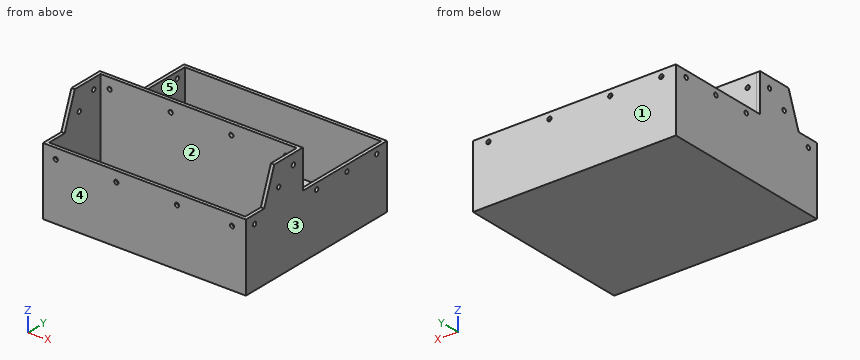
```python
from build123d import *

# Parameters (mm, degrees)
SKETCH1_W           = 190.5
SKETCH1_H           = 166.116
BOSS_EXTRUDE1_DEPTH = 95.25
CUT_EXTRUDE1_DEPTH  = 92.075
CUT_EXTRUDE5_DEPTH  = 35.98418
SKETCH17_W          = 190.5
SKETCH17_H          = 33.474363619
CUT_EXTRUDE6_DEPTH  = 31.75
BOSS_EXTRUDE8_DEPTH = 190.5
SKETCH19_W          = 184.15
SKETCH19_H          = 30.313503047
CUT_EXTRUDE7_DEPTH  = 92.075
SKETCH20_W          = 184.15
SKETCH20_H          = 33.914711244
CUT_EXTRUDE8_DEPTH  = 13.175
CUT_EXTRUDE9_DEPTH  = 60.325
SKETCH23_R          = 2.00000108
CUT_EXTRUDE10_DEPTH = 2.54
SKETCH24_R          = 2
SKETCH24_R_2        = 2.00000108
CUT_EXTRUDE11_DEPTH = 2.54
SKETCH25_R          = 2.00000108
CUT_EXTRUDE12_DEPTH = 229.607619873
SKETCH27_R          = 2.00000108
CUT_EXTRUDE13_DEPTH = 3.175
SKETCH28_R          = 2.00000108
CUT_EXTRUDE15_DEPTH = 229.607619873


with BuildPart() as part:
    # Sketch1 → Boss-Extrude1 (new body)
    with BuildSketch(Plane.XY):
        Rectangle(SKETCH1_W, SKETCH1_H)
    extrude(amount=BOSS_EXTRUDE1_DEPTH)

    # Sketch3 → Cut-Extrude1 (cut)
    with BuildSketch(Plane.XY.offset(95.25)):
        Polygon((-92.075, 79.883), (-92.075, 32.891702926), (-92.075, -16.095133334), (92.075, -16.095133334), (92.075, 48.662739539), (92.075, 79.883), (83.88326961, 79.883), (-81.085829842, 79.883), align=None)
    extrude(amount=-CUT_EXTRUDE1_DEPTH, mode=Mode.SUBTRACT)

    # Sketch15 → Cut-Extrude5 (cut)
    with BuildSketch(Plane.XY.offset(95.25)):
        Polygon((95.25, -16.109272762), (95.25, 83.058), (-95.25, 83.058), (-95.25, -16.109272762), (-92.075, -16.095133334), (-92.075, 79.883), (92.075, 79.883), (92.075, -16.095133334), align=None)
    extrude(amount=-CUT_EXTRUDE5_DEPTH, mode=Mode.SUBTRACT)

    # Sketch17 → Cut-Extrude6 (cut)
    with BuildSketch(Plane.XY.offset(95.25)):
        with Locations((0, -66.320818191)):
            Rectangle(SKETCH17_W, SKETCH17_H)
    extrude(amount=-CUT_EXTRUDE6_DEPTH, mode=Mode.SUBTRACT)

    # Sketch18 → Boss-Extrude8 (add)
    with BuildSketch(Plane.ZY.offset(95.25)):
        Polygon((63.5, -49.583636381), (63.5, -61.506100001), (95.25, -49.583636381), align=None)
    extrude(amount=-BOSS_EXTRUDE8_DEPTH)

    # Sketch19 → Cut-Extrude7 (cut)
    with BuildSketch(Plane.XY.offset(95.25)):
        with Locations((0, -34.426884857)):
            Rectangle(SKETCH19_W, SKETCH19_H)
    extrude(amount=-CUT_EXTRUDE7_DEPTH, mode=Mode.SUBTRACT)

    # Sketch20 → Cut-Extrude8 (cut)
    with BuildSketch(Plane(origin=(0, -74.803163357, 28.08938563), x_dir=(1, 0, 0), z_dir=(0, -0.9361719099317519, 0.3515425366221503))):
        with Locations((0, 54.782261491)):
            Rectangle(SKETCH20_W, SKETCH20_H)
    extrude(amount=-CUT_EXTRUDE8_DEPTH, mode=Mode.SUBTRACT)

    # Sketch21 → Cut-Extrude9 (cut)
    with BuildSketch(Plane.XY.offset(63.5)):
        Polygon((-92.075, -61.506100001), (-92.075, -49.583636381), (92.075, -49.583636381), (92.075, -61.506100001), (92.075, -79.883), (-92.075, -79.883), align=None)
    extrude(amount=-CUT_EXTRUDE9_DEPTH, mode=Mode.SUBTRACT)

    # Sketch23 → Cut-Extrude10 (cut)
    with BuildSketch(Plane.XZ.offset(83.058)):
        with Locations(Location((-83.319719804, 53.848, 0), (0, 0, 270))):
            Circle(SKETCH23_R)
        with Locations(Location((-26.423719804, 53.848, 0), (0, 0, 270))):
            Circle(SKETCH23_R)
        with Locations(Location((30.472280196, 53.848, 0), (0, 0, 270))):
            Circle(SKETCH23_R)
        with Locations(Location((82.288280196, 53.848, 0), (0, 0, 270))):
            Circle(SKETCH23_R)
    extrude(amount=-CUT_EXTRUDE10_DEPTH, mode=Mode.SUBTRACT)

    # Sketch24 → Cut-Extrude11 (cut)
    with BuildSketch(Plane(origin=(0, 83.058, 0), x_dir=(1, 0, 0), z_dir=(0, 1, 0))):
        with Locations(Location((80.65616897, -53.55082, 0), (0, 0, 270))):
            Circle(SKETCH24_R)
        with Locations(Location((23.50616897, -53.55082, 0), (0, 0, 270))):
            Circle(SKETCH24_R_2)
        with Locations(Location((-33.64383103, -53.55082, 0), (0, 0, 270))):
            Circle(SKETCH24_R_2)
        with Locations(Location((-81.568772043, -53.55082, 0), (0, 0, 270))):
            Circle(SKETCH24_R_2)
    extrude(amount=-CUT_EXTRUDE11_DEPTH, mode=Mode.SUBTRACT)

    # Sketch25 → Cut-Extrude12 (cut, through all)
    with BuildSketch(Plane(origin=(95.25, 0, 0), x_dir=(0, 0, -1), z_dir=(1, 0, 0))):
        with Locations((-53.42382, 70.993)):
            Circle(SKETCH25_R)
        with Locations((-53.42382, 35.941)):
            Circle(SKETCH25_R)
        with Locations((-53.42382, 0.217760577)):
            Circle(SKETCH25_R)
    extrude(amount=-CUT_EXTRUDE12_DEPTH, mode=Mode.SUBTRACT)

    # Sketch27 → Cut-Extrude13 (cut)
    with BuildSketch(Plane(origin=(0, -16.095133334, 0), x_dir=(1, 0, 0), z_dir=(0, 1, 0))):
        with Locations(Location((82.042, -85.344, 0), (0, 0, 270))):
            Circle(SKETCH27_R)
        with Locations(Location((30.734, -85.344, 0), (0, 0, 270))):
            Circle(SKETCH27_R)
        with Locations(Location((-26.268567804, -85.344, 0), (0, 0, 270))):
            Circle(SKETCH27_R)
        with Locations(Location((-83.566, -85.344, 0), (0, 0, 270))):
            Circle(SKETCH27_R)
    extrude(amount=-CUT_EXTRUDE13_DEPTH, mode=Mode.SUBTRACT)

    # Sketch28 → Cut-Extrude15 (cut, through all)
    with BuildSketch(Plane(origin=(95.25, 0, 0), x_dir=(0, 0, -1), z_dir=(1, 0, 0))):
        with Locations((-55.372, -72.898)):
            Circle(SKETCH28_R)
        with Locations((-74.422, -44.381878841)):
            Circle(SKETCH28_R)
        with Locations((-85.598, -27.204003713)):
            Circle(SKETCH28_R)
    extrude(amount=-CUT_EXTRUDE15_DEPTH, mode=Mode.SUBTRACT)


solid = part.part
```
Geometry check sheet. Reference: the model listing, model coordinates, mm. Face numbers are marked on the shaded views. A direction names the side the tool comes from. Coordinates: 2 decimals unless noted, no trailing zeros. Write each loop counter-clockwise with the first axis right and the second up, starting at its lowest first coordinate (ties: lowest second). Pieces come first, ordered by that corner, then holes. Notation, with made-up numbers: (48, 25) -> (102, 25) arc R34 cw to (102, 55) -> close; hole circle Ø1 at (-8.5, -4). An arc over 180 degrees is marked (long way). Use CSV: the item, a comma, the result in double quotes. Start each with the question number.
Item 1: Thickness scan on line 1 (Y direction, x = 75.5, z = 23); line 2 (Y direction, x = 82.5, z = 59.5); line 3 (X direction, y = -48.5, z = 4) (3 decimals). Record the ranges inside material, lowest first.
Item 2: Cross-section at A-A, the plane z = 15. Record the cut outline in (x, y) (3 decimals).
Item 3: Cross-section at B-B, the plane x = 71.5. Record the cut outline in (y, z) (3 decimals), plus the area to 3 significant figures.
Item 4: Cross-section at D-D, the plane z = 68.5. Record the cut outline in (x, y) (3 decimals), plus the area to 3 significant figures.
Item 5: Mould release check, pull along X, two halves, no side actions. Record for the marked faces 3, 4 and 5: released by +X, released by -X, zero draft, split by the parting line, or undercut.
Item 6: Cross-section at C-C, the plane y = 27. Record the cut outline in (x, z) (3 decimals).
Item 7: Set-up check for the marked faces 1 and 2: record each of +Z, -Z, +X, -X, +Y, -Y from which the full face is reachable in a straight line by a thin tool's end or side.
Item 8: Depth check by flat-ended pin: pin 1 Ø3.5 at (y, z) = (-27.2, 85.6) entering from -X; pin 2 Ø5 at (y, z) = (35.94, 53.42) entering from +X; pin 3 Ø23.5 at (x, y) = (12, -76.5) entering from +Z; pin 4 Ø4 at (x, y) = (-60, 38.5) entering from +Z (3 decimals). Enter the tip coordinate at first touch or a pass-through.
Answers:
1,line 1,"-83.06 to -79.88, -19.27 to -16.1, 79.88 to 83.06"
1,line 2,"-83.06 to -79.88, -19.27 to -16.1"
1,line 3,"-95.25 to -92.075, 92.075 to 95.25"
2,outline,"(-95.25, -83.058) -> (95.25, -83.058) -> (95.25, 83.058) -> (-95.25, 83.058) -> close; hole (-92.075, -79.883) -> (92.075, -79.883) -> (92.075, -19.27) -> (-92.075, -19.27) -> close; hole (-92.075, -16.095) -> (92.075, -16.095) -> (92.075, 79.883) -> (-92.075, 79.883) -> close"
3,outline,"(-83.058, 0) -> (83.058, 0) -> (83.058, 59.266) -> (79.883, 59.266) -> (79.883, 3.175) -> (-16.095, 3.175) -> (-16.095, 95.25) -> (-19.27, 95.25) -> (-19.27, 3.175) -> (-79.883, 3.175) -> (-79.883, 63.5) -> (-83.058, 63.5) -> close"
3,area,"1,190 mm^2"
4,outline,"(-95.25, -59.629) -> (-92.075, -59.629) -> (-92.075, -19.27) -> (92.075, -19.27) -> (92.075, -59.629) -> (95.25, -59.629) -> (95.25, -16.109) -> (92.075, -16.095) -> (-92.075, -16.095) -> (-95.25, -16.109) -> close"
4,area,"861 mm^2"
5,face 3,"released by +X"
5,face 4,"zero draft"
5,face 5,"undercut"
6,outline,"(-95.25, 0) -> (95.25, 0) -> (95.25, 59.266) -> (92.075, 59.266) -> (92.075, 3.175) -> (-92.075, 3.175) -> (-92.075, 59.266) -> (-95.25, 59.266) -> close"
7,face 1,"+Z, -Z, +X, -X, +Y"
7,face 2,"+Z"
8,pin 1,"through"
8,pin 2,"x = 95.25"
8,pin 3,"z = 63.5"
8,pin 4,"z = 3.175"
